Autodesk Inventor part; units mm, degrees
ref_plane "YZ Plane" through (0, 0, 0) normal (1, 0, 0) x (0, 1, 0)
ref_plane "XZ Plane" through (0, 0, 0) normal (0, 1, 0) x (-1, 0, 0)
ref_plane "XY Plane" through (0, 0, 0) normal (0, 0, 1) x (1, 0, 0)
sketch "Sketch1" plane through (0, 0, 0) normal (0, 0, 1) x (1, 0, 0)
  arc A0 (8, 0) -> (-8, 0) centre (0, 0) ccw
  arc A1 (15, 0) -> (-15, 0) centre (0, 0) ccw
  line L0 (-8, 0) -> (-15, 0)
  line L1 (-15, 0) -> (-20, 0)
  line L2 (-20, 0) -> (-20, 5)
  line L3 (-20, 5) -> (-14.1421, 5)
  line L4 (8, 0) -> (15, 0)
  line L5 (15, 0) -> (20, 0)
  line L6 (20, 0) -> (20, 5)
  line L7 (20, 5) -> (14.1421, 5)
  dimension "d0" = 16
  dimension "d1" = 30
  dimension "d2" = 5
  dimension "d3" = 5
  dimension "d4" = 5
  dimension "d5" = 5
extrude "Extrusion1" add sketch "Sketch1" along normal blind 15
sketch "Sketch2" plane through (8, 0, 0) normal (0, -1, 0) x (1, 0, 0)
  line L0 (-28, 0) -> (-28, 15)
  line L1 (-28, 7.5) -> (-24, 7.5)
  line L2 (12, 0) -> (12, 15)
  line L3 (12, 7.5) -> (8, 7.5)
  circle A0 centre (-24, 7.5) radius 1.75
  circle A1 centre (8, 7.5) radius 1.75
  point P0 (-8, 0)
  dimension "d8" = 4
  dimension "d9" = 4
  dimension "d10" = 3.5
  dimension "d11" = 3.5
extrude "Extrusion2" cut sketch "Sketch2" against normal through all
properties part number "prism_holder_2"
Model file for the job. Use its own axes, mm. A direction names the side the tool comes from. Coordinates: 2 decimals unless noted, no trailing zeros. Order: outer loops, then holes, each group sorted by start corner. A loop starts at its lowest first (then second) coordinate and runs counter-clockwise, first axis right, second up. Notation, with made-up numbers: M -32,-27.5 L -6,-27.5 A20 cw -6,10.5 Z; hole C -14.75,78 d10. An arc over 180 degrees is marked long. Answer as CSV lines item,"result".
(1) Wall check: line 1 along Z through (x, y) = (-16, 3.6); line 2 along X through (y, z) = (3, 1.5); line 3 along Y through (x, z) = (0, 6.75). Give the ranges that are in metal, low to high.
Geometry says:
line 1,"z = 0 to 5.75, 9.25 to 15"
line 2,"x = -20 to -7.42, 7.42 to 20"
line 3,"y = 8 to 15"
(2) Band-saw the part on C-C, the plane z = 7.5. List the corners of the cut face in (x, y).
Geometry says:
outline,"M -20,0 L -17.75,0 L -17.75,5 L -20,5 Z; M -14.25,0 L -8,0 A8 cw 8,0 L 14.25,0 L 14.25,5 L 14.14,5 A15 ccw -14.14,5 L -14.25,5 Z; M 17.75,0 L 20,0 L 20,5 L 17.75,5 Z"
(3) Pull direction Z, two halves, no side cores. Call faces 1 (the cylindrical face through (-14.383, 2.465, 6.83)), 2 (the flat face through (0, 9, 15)), 3 (the flat face through (0, 9, 0)): +Z half, -Z half, draft (parallel to the pull), parting line (faces both ways), or undercut.
Geometry says:
face 1,"undercut"
face 2,"+Z half"
face 3,"-Z half"
(4) Flat gauge pins, fed straight in: pin 1 (1.8 mm diameter, centred on x = -17, z = 4.5, fed in from +Y); pin 2 (1 mm diameter, centred on y = 8, z = 8, fed in from -X); pin 3 (2 mm diameter, centred on x = 11.5, z = 2.5, fed in from +Y). Where does each tip first touch, or does it go through?
Geometry says:
pin 1,"stops at y = 5"
pin 2,"stops at x = -12.99"
pin 3,"stops at y = 10.71"
(5) Band-saw the part on B-B, the plane y = 2.25. List the corners of the cut face in (x, z).
Geometry says:
outline,"M -20,0 L -7.68,0 L -7.68,15 L -20,15 Z; M 7.68,0 L 20,0 L 20,15 L 7.68,15 Z; hole C -16,7.5 d3.5; hole C 16,7.5 d3.5"
(6) Band-saw the part on A-A, the plane x = 16. List the corners of the cut face in (y, z).
Geometry says:
outline,"M 0,0 L 5,0 L 5,5.75 L 0,5.75 Z; M 0,9.25 L 5,9.25 L 5,15 L 0,15 Z"
(7) 3-axis set-ups, long thin cutter, end or side, ignore diameter. For faces 4 (the cylindrical face through (0, 8, 7)), 5 (the flat face through (18, 5, 7)), 6 (the flat face through (-18, 5, 7)): which of +Z, -Z, +X, -X, +Y, -Y reach the whole face in a straight line?
Geometry says:
face 4,"+Z, -Z, -Y"
face 5,"+Z, -Z, +X, +Y"
face 6,"+Z, -Z, -X, +Y"
(8) Band-saw the part on D-D, the plane z = 10.5. List the corners of the cut face in (x, y).
Geometry says:
outline,"M -20,0 L -8,0 A8 cw 8,0 L 20,0 L 20,5 L 14.14,5 A15 ccw -14.14,5 L -20,5 Z"
